from build123d import *

# Parameters (mm, degrees)
EXTRUDE_1_DEPTH     = 2
EXTRUDE_2_DEPTH     = 1.5
EXTRUDE_2_TAPER     = 30
CUT_EXTRUDE_1_REACH = 95.039
SKETCH_3_R          = 1.131038805


with BuildPart() as part:
    # 草图1 → 凸台-拉伸1 (new body)
    with BuildSketch(Plane(origin=(0, 0, 0), x_dir=(1, 0, 0), z_dir=(0, 1, 0))):
        with BuildLine():
            Line((-65.314374304, 18.3), (-88.142801429, 18.3))
            ThreePointArc((-88.142801429, 18.3), (-89.450948974, 17.758147545), (-89.992801429, 16.45))
            Line((-89.992801429, 16.45), (-89.992801429, -6.378427125))
            ThreePointArc((-89.992801429, -6.378427125), (-89.450948974, -7.68657467), (-88.142801429, -8.228427125))
            Line((-88.142801429, -8.228427125), (-70.142801429, -8.228427125))
            ThreePointArc((-70.142801429, -8.228427125), (-69.434837079, -8.08760426), (-68.834653884, -7.68657467))
            Line((-68.834653884, -7.68657467), (-64.006226759, -2.858147545))
            ThreePointArc((-64.006226759, -2.858147545), (-63.605197169, -2.25796435), (-63.464374304, -1.55))
            Line((-63.464374304, -1.55), (-63.464374304, 16.45))
            ThreePointArc((-63.464374304, 16.45), (-64.006226759, 17.758147545), (-65.314374304, 18.3))
        make_face()
        with BuildLine():
            Line((-65.314374304, 17.3), (-88.142801429, 17.3))
            ThreePointArc((-88.142801429, 17.3), (-88.743842193, 17.051040764), (-88.992801429, 16.45))
            Line((-88.992801429, 16.45), (-88.992801429, -6.378427125))
            ThreePointArc((-88.992801429, -6.378427125), (-88.743842193, -6.979467889), (-88.142801429, -7.228427125))
            Line((-88.142801429, -7.228427125), (-70.142801429, -7.228427125))
            ThreePointArc((-70.142801429, -7.228427125), (-69.817520511, -7.163724728), (-69.541760665, -6.979467889))
            Line((-69.541760665, -6.979467889), (-64.71333354, -2.151040764))
            ThreePointArc((-64.71333354, -2.151040764), (-64.529076702, -1.875280918), (-64.464374304, -1.55))
            Line((-64.464374304, -1.55), (-64.464374304, 16.45))
            ThreePointArc((-64.464374304, 16.45), (-64.71333354, 17.051040764), (-65.314374304, 17.3))
        make_face(mode=Mode.SUBTRACT)
    extrude(amount=-EXTRUDE_1_DEPTH)

    # 草图2 → 凸台-拉伸2 (add)
    with BuildSketch(Plane(origin=(0, 0, 0), x_dir=(1, 0, 0), z_dir=(0, 1, 0))):
        with BuildLine():
            Line((-65.314374304, 19.3), (-88.142801429, 19.3))
            ThreePointArc((-88.142801429, 19.3), (-90.158055755, 18.465254326), (-90.992801429, 16.45))
            Line((-90.992801429, 16.45), (-90.992801429, -6.378427125))
            ThreePointArc((-90.992801429, -6.378427125), (-90.158055755, -8.393681451), (-88.142801429, -9.228427125))
            Line((-88.142801429, -9.228427125), (-70.142801429, -9.228427125))
            ThreePointArc((-70.142801429, -9.228427125), (-69.052153647, -9.011483793), (-68.127547103, -8.393681451))
            Line((-68.127547103, -8.393681451), (-63.299119978, -3.565254327))
            ThreePointArc((-63.299119978, -3.565254327), (-62.681317637, -2.640647782), (-62.464374304, -1.55))
            Line((-62.464374304, -1.55), (-62.464374304, 16.45))
            ThreePointArc((-62.464374304, 16.45), (-63.299119978, 18.465254326), (-65.314374304, 19.3))
        make_face()
    extrude(amount=EXTRUDE_2_DEPTH, taper=EXTRUDE_2_TAPER)

    # 草图3 → 切除-拉伸1 (cut, up to next)
    with BuildSketch(Plane.XZ, mode=Mode.PRIVATE) as cut_extrude_1_sk1:
        with Locations(Location((-86.712801429, -15.02, 0), (0, 0, 270))):
            Circle(SKETCH_3_R)
    cut_extrude_1_tool1 = extrude(cut_extrude_1_sk1.sketch, amount=-CUT_EXTRUDE_1_REACH, mode=Mode.PRIVATE) & part.part
    # 草图3 → 切除-拉伸1 (cut, up to next)
    with BuildSketch(Plane.XZ, mode=Mode.PRIVATE) as cut_extrude_1_sk2:
        with BuildLine():
            Line((-85.91303622, -9.251807666), (-80.944609096, -14.220234791))
            ThreePointArc((-80.944609096, -14.220234791), (-80.944609096, -15.819765208), (-82.544139513, -15.819765208))
            Line((-82.544139513, -15.819765208), (-87.512566638, -10.851338084))
            ThreePointArc((-87.512566638, -10.851338084), (-87.512566638, -9.251807666), (-85.91303622, -9.251807666))
        make_face()
    cut_extrude_1_tool2 = extrude(cut_extrude_1_sk2.sketch, amount=-CUT_EXTRUDE_1_REACH, mode=Mode.PRIVATE) & part.part
    # 草图3 → 切除-拉伸1 (cut, up to next)
    with BuildSketch(Plane.XZ, mode=Mode.PRIVATE) as cut_extrude_1_sk3:
        with BuildLine():
            Line((-70.91303622, 5.748192334), (-65.944609096, 0.779765209))
            ThreePointArc((-65.944609096, 0.779765209), (-65.944609096, -0.819765208), (-67.544139513, -0.819765208))
            Line((-67.544139513, -0.819765208), (-72.512566638, 4.148661916))
            ThreePointArc((-72.512566638, 4.148661916), (-72.512566638, 5.748192334), (-70.91303622, 5.748192334))
        make_face()
    cut_extrude_1_tool3 = extrude(cut_extrude_1_sk3.sketch, amount=-CUT_EXTRUDE_1_REACH, mode=Mode.PRIVATE) & part.part
    # 草图3 → 切除-拉伸1 (cut, up to next)
    with BuildSketch(Plane.XZ, mode=Mode.PRIVATE) as cut_extrude_1_sk4:
        with BuildLine():
            Line((-75.91303622, 5.748192334), (-65.944609096, -4.220234791))
            ThreePointArc((-65.944609096, -4.220234791), (-65.944609096, -5.819765208), (-67.544139513, -5.819765208))
            Line((-67.544139513, -5.819765208), (-77.512566638, 4.148661916))
            ThreePointArc((-77.512566638, 4.148661916), (-77.512566638, 5.748192334), (-75.91303622, 5.748192334))
        make_face()
    cut_extrude_1_tool4 = extrude(cut_extrude_1_sk4.sketch, amount=-CUT_EXTRUDE_1_REACH, mode=Mode.PRIVATE) & part.part
    # 草图3 → 切除-拉伸1 (cut, up to next)
    with BuildSketch(Plane.XZ, mode=Mode.PRIVATE) as cut_extrude_1_sk5:
        with BuildLine():
            Line((-80.91303622, 5.748192334), (-65.944609096, -9.220234791))
            ThreePointArc((-65.944609096, -9.220234791), (-65.944609096, -10.819765208), (-67.544139513, -10.819765208))
            Line((-67.544139513, -10.819765208), (-82.512566638, 4.148661916))
            ThreePointArc((-82.512566638, 4.148661916), (-82.512566638, 5.748192334), (-80.91303622, 5.748192334))
        make_face()
    cut_extrude_1_tool5 = extrude(cut_extrude_1_sk5.sketch, amount=-CUT_EXTRUDE_1_REACH, mode=Mode.PRIVATE) & part.part
    # 草图3 → 切除-拉伸1 (cut, up to next)
    with BuildSketch(Plane.XZ, mode=Mode.PRIVATE) as cut_extrude_1_sk6:
        with BuildLine():
            Line((-85.91303622, 0.748192334), (-70.944609096, -14.220234791))
            ThreePointArc((-70.944609096, -14.220234791), (-70.944609096, -15.819765208), (-72.544139513, -15.819765208))
            Line((-72.544139513, -15.819765208), (-87.512566638, -0.851338084))
            ThreePointArc((-87.512566638, -0.851338084), (-87.512566638, 0.748192334), (-85.91303622, 0.748192334))
        make_face()
    cut_extrude_1_tool6 = extrude(cut_extrude_1_sk6.sketch, amount=-CUT_EXTRUDE_1_REACH, mode=Mode.PRIVATE) & part.part
    # 草图3 → 切除-拉伸1 (cut, up to next)
    with BuildSketch(Plane.XZ, mode=Mode.PRIVATE) as cut_extrude_1_sk7:
        with BuildLine():
            Line((-85.91303622, 5.748192334), (-65.944609096, -14.220234791))
            ThreePointArc((-65.944609096, -14.220234791), (-65.944609096, -15.819765208), (-67.544139513, -15.819765208))
            Line((-67.544139513, -15.819765208), (-87.512566638, 4.148661916))
            ThreePointArc((-87.512566638, 4.148661916), (-87.512566638, 5.748192334), (-85.91303622, 5.748192334))
        make_face()
    cut_extrude_1_tool7 = extrude(cut_extrude_1_sk7.sketch, amount=-CUT_EXTRUDE_1_REACH, mode=Mode.PRIVATE) & part.part
    # 草图3 → 切除-拉伸1 (cut, up to next)
    with BuildSketch(Plane.XZ, mode=Mode.PRIVATE) as cut_extrude_1_sk8:
        with BuildLine():
            Line((-85.91303622, -4.251807666), (-75.944609096, -14.220234791))
            ThreePointArc((-75.944609096, -14.220234791), (-75.944609096, -15.819765208), (-77.544139513, -15.819765208))
            Line((-77.544139513, -15.819765208), (-87.512566638, -5.851338084))
            ThreePointArc((-87.512566638, -5.851338084), (-87.512566638, -4.251807666), (-85.91303622, -4.251807666))
        make_face()
    cut_extrude_1_tool8 = extrude(cut_extrude_1_sk8.sketch, amount=-CUT_EXTRUDE_1_REACH, mode=Mode.PRIVATE) & part.part
    add(cut_extrude_1_tool1.solids().sort_by_distance((-86.712801, 0, -15.02))[0], mode=Mode.SUBTRACT)
    add(cut_extrude_1_tool2.solids().sort_by_distance((-84.228588, 0, -12.535786))[0], mode=Mode.SUBTRACT)
    add(cut_extrude_1_tool3.solids().sort_by_distance((-69.228588, 0, 2.464214))[0], mode=Mode.SUBTRACT)
    add(cut_extrude_1_tool4.solids().sort_by_distance((-71.728588, 0, -0.035786))[0], mode=Mode.SUBTRACT)
    add(cut_extrude_1_tool5.solids().sort_by_distance((-74.228588, 0, -2.535786))[0], mode=Mode.SUBTRACT)
    add(cut_extrude_1_tool6.solids().sort_by_distance((-79.228588, 0, -7.535786))[0], mode=Mode.SUBTRACT)
    add(cut_extrude_1_tool7.solids().sort_by_distance((-76.728588, 0, -5.035786))[0], mode=Mode.SUBTRACT)
    add(cut_extrude_1_tool8.solids().sort_by_distance((-81.728588, 0, -10.035786))[0], mode=Mode.SUBTRACT)


solid = part.part
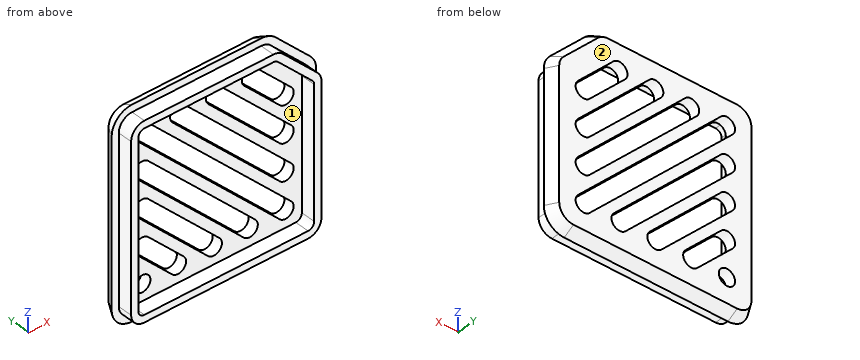
Design review of the part built by this model. Coordinates are the model's own, in mm. Face numbers are marked on the shaded views. Round coordinates to 2 decimals unless told otherwise and drop trailing zeros. Write each loop counter-clockwise with the first axis right and the second up, starting at its lowest first coordinate (ties: lowest second). Pieces come first, ordered by that corner, then holes. Notation, with made-up numbers: M -36.75,75.5 L -4.75,75.5 A24 ccw -4.75,97.5 Z; hole C 59,74 d9. An arc over 180 degrees is marked long. One line per item, written item: value. Start each with the question number.
1. To check wall thickness, follow probe 1 along X at (y, z) = (1.1, -15.02); probe 2 along X at (y, z) = (0.6, -1.75); probe 3 along X at (y, z) = (0.7, -15.02). State the ranges of each line that lie inside material, in increasing order. Write a range as from..to.
2. Take a section at A-A on y = -0.5. State the section outline as (x, z) points.
3. Take a section at B-B on z = -15.02. State how many separate pieces and enclosed holes the cut face has, then the cut area to 3 significant figures.
4. Draft analysis for pull direction X (two halves, no side actions). For the marked faces 1 and 2, state which applies: pulls with the +X half, pulls with the -X half, needs draft (parallel to the pull), parting line crosses it, or undercut.
5. Clearance check with flat-ended pins moving along their axes: P1, Ø0.6, axis at y = -1, z = -4.5, coming from the -X side; P2, Ø1.5, axis at x = -71, z = -4.5, coming from the -Y side; P3, Ø1.6, axis at x = -77, y = -1, coming from the +Z side. State where each tip first meets the part, or that it passes through.
Computed:
1. probe 1: x = -90.36..-87.84, -85.58..-83.34, -80.61..-78.34, -75.61..-73.34, -70.61..-68.34, -65.61..-63.1
1. probe 2: x = -90.65..-86.61, -83.41..-81.61, -78.41..-76.61, -73.41..-71.61, -68.41..-62.81
1. probe 3: x = -90.59..-87.84, -85.58..-83.34, -80.61..-78.34, -75.61..-73.34, -70.61..-68.34, -65.61..-62.87
2. outline: M -89.99,-16.45 A1.85 ccw -88.14,-18.3 L -65.31,-18.3 A1.85 ccw -63.46,-16.45 L -63.46,1.55 A1.85 ccw -64.01,2.86 L -68.83,7.69 A1.85 ccw -70.14,8.23 L -88.14,8.23 A1.85 ccw -89.99,6.38 Z; hole M -88.99,-16.45 A0.85 ccw -88.14,-17.3 L -65.31,-17.3 A0.85 ccw -64.46,-16.45 L -64.46,1.55 A0.85 ccw -64.71,2.15 L -69.54,6.98 A0.85 ccw -70.14,7.23 L -88.14,7.23 A0.85 ccw -88.99,6.38 Z
3. separate pieces: 6
3. enclosed holes: 0
3. area: 25.7 mm²
4. face 1: undercut
4. face 2: needs draft
5. P1: stops at x = -89.99
5. P2: stops at y = 0
5. P3: stops at z = 8.23
